The listing builds one solid part. Answer for the finished solid, in the listing's coordinates (mm). Round coordinates to 2 decimals unless told otherwise and drop trailing zeros. Write each loop counter-clockwise with the first axis right and the second up, starting at its lowest first coordinate (ties: lowest second). Pieces come first, ordered by that corner, then holes.
(1) A cutting plane is placed at A-A, the plane x = 0. Give the vertices of the cut face in (y, z) (3 decimals).
(2) A cutting plane is placed at C-C, the plane x = 3. Give the vertices of the cut face in (y, z).
(3) A cutting plane is placed at B-B, the plane y = 0.25. Give the vertices of the cut face in (x, z) (3 decimals).
(4) The mould has two halves that part along Z. Classify faces 1 (the face through (-0.271, 0.014, 21.745)), 2 (the face through (-7.965, 0, 0)), 3 (the face through (0, 0, -30)): +Z half, -Z half, draft (parallel to the pull), parting line (faces both ways), or undercut.
(5) This flat-tipped pin is pushed along its axis until it touches: pin 1 Ø2 at (x, z) = (3, 31.64) entering from -Y. Where does it stop, or does it pass through?
(6) Find the intervals of material crossed by probe 1 along Z at (x, y) = (0, -0.1) (3 decimals); probe 2 along Z at (x, y) = (-3.25, -0.6); probe 3 along Z at (x, y) = (6.75, 0.1), in increasing order.
from build123d import *

# Parameters (mm, degrees)
F0_R     = 1.25
F1_DEPTH = 1


with BuildPart() as f1:
    # F0 (on Front) → F1 (new body, symmetric)
    with BuildSketch(Plane.XZ):
        with BuildLine():
            Line((-7.965, 30), (-7.965, -30))
            Line((-7.965, -30), (7.965, -30))
            Line((7.965, -30), (7.965, 30))
            ThreePointArc((7.965, 30), (0, 37.965), (-7.965, 30))
        make_face()
        with Locations((-3, 31.640445)):
            Circle(F0_R, mode=Mode.SUBTRACT)
        with Locations((0, 22.965)):
            Circle(F0_R, mode=Mode.SUBTRACT)
        with Locations((3, 31.640445)):
            Circle(F0_R, mode=Mode.SUBTRACT)
    extrude(amount=F1_DEPTH, both=True)


solid = f1.part
Solutions:
1. outline: (-1, -30) - (1, -30) - (1, 21.715) - (-1, 21.715) - close; (-1, 24.215) - (1, 24.215) - (1, 37.965) - (-1, 37.965) - close
2. outline: (-1, -30) - (1, -30) - (1, 30.39) - (-1, 30.39) - close; (-1, 32.89) - (1, 32.89) - (1, 37.38) - (-1, 37.38) - close
3. outline: (-7.965, -30) - (7.965, -30) - (7.965, 30) arc R7.965 ccw to (-7.965, 30) - close; hole circle Ø2.5 at (-3, 31.64); hole circle Ø2.5 at (0, 22.965); hole circle Ø2.5 at (3, 31.64)
4. face 1: undercut
4. face 2: draft
4. face 3: -Z half
5. pin 1: passes through
6. probe 1: z = -30 to 21.715, 24.215 to 37.965
6. probe 2: z = -30 to 30.42, 32.87 to 37.27
6. probe 3: z = -30 to 34.23
